Autodesk Fusion 360 part; units mm, degrees
sketch "Sketch1" plane through (0, 0, 0) normal (0, 1, 0) x (1, 0, 0)
  line L0 (20, 0) -> (40, 0)
  line L1 (40, 0) -> (40, -15)
  line L2 (26, -45) -> (0, -45)
  line L3 (-26, -45) -> (0, -45)
  line L4 (-40, 0) -> (-40, -15)
  line L5 (-20, 0) -> (-40, 0)
  line L6 (20, -20) -> (-20, -20)
  line L7 (-20, -20) -> (-20, 0)
  line L8 (20, 0) -> (20, -20)
  line L9 (-40, 0) -> (-40, -15)
  line L10 (0, -45) -> (-26, -45)
  line L11 (-40, -15) -> (-26, -45)
  line L12 (40, -15) -> (26, -45)
  dimension "d5" = 15
  dimension "d6" = 26
extrude "Extrude1" add sketch "Sketch1" along normal mid plane 60
sketch "Sketch3" plane through (0, 0, 0) normal (1, 0, 0) x (0, 1, 0)
  line L0 (-30, 45) -> (-21, 45)
  line L1 (-21, 45) -> (-21, 30)
  line L2 (-21, 30) -> (-30, 30)
  line L3 (-30, 30) -> (-30, 45)
  line L4 (21, 45) -> (21, 30)
  line L5 (21, 30) -> (30, 30)
  line L6 (30, 30) -> (30, 45)
  line L7 (30, 45) -> (21, 45)
  dimension "d9" = 9
  dimension "d10" = 15
extrude "Extrude2" cut sketch "Sketch3" along normal mid plane 120
sketch "Sketch4" plane through (0, 0, 45) normal (0, 0, 1) x (-1, 0, 0)
  line L0 (-26, -21) -> (26, -21)
  line L1 (26, -21) -> (26, 21)
  line L2 (26, 21) -> (-26, 21)
  line L3 (-26, 21) -> (-26, -21)
  line L4 (40, 30) -> (40, 15)
  line L5 (40, 15) -> (50, 15)
  line L6 (50, 15) -> (50, -15)
  line L7 (50, -15) -> (40, -15)
  line L8 (40, -15) -> (28, -15)
  line L9 (28, -15) -> (28, 15)
  line L10 (28, 15) -> (40, 15)
  line L11 (-50, 15) -> (-50, -15)
  line L12 (-50, -15) -> (-40, -15)
  line L13 (-40, -15) -> (-28, -15)
  line L14 (-28, -15) -> (-28, 15)
  line L15 (-28, 15) -> (-40, 15)
  line L16 (-40, 15) -> (-50, 15)
  dimension "d13" = 15
  dimension "d14" = 10
  dimension "d15" = 30
extrude "Extrude3" add sketch "Sketch4" along normal blind 28 from surface at -45 contours L5 L6 L7 L8 L9 L10 | L11 L12 L13 L14 L15 L16
sketch "Sketch5" plane through (0, 0, 45) normal (0, 0, 1) x (-1, 0, 0)
  line L0 (-26, -21) -> (26, -21)
  line L1 (26, -21) -> (26, 21)
  line L2 (26, 21) -> (-26, 21)
  line L3 (-26, 21) -> (-26, -21)
  circle A0 centre (0, 0) radius 15
  dimension "d19" = 30
extrude "Extrude4" add sketch "Sketch5" along normal blind 30 contours A0
sketch "Sketch6" plane through (0, 0, 0) normal (0, 1, 0) x (-1, 0, 0)
  line L0 (-10, 55) -> (-10, 65)
  line L1 (-10, 55) -> (-18, 55)
  line L2 (-18, 55) -> (-18, 65)
  line L3 (-18, 65) -> (-10, 65)
  line L4 (-10, 65) -> (-10, 55)
  line L5 (18, 55) -> (18, 65)
  line L6 (10, 55) -> (18, 55)
  line L7 (10, 65) -> (10, 55)
  line L8 (18, 65) -> (10, 65)
extrude "Extrude5" cut sketch "Sketch6" along normal mid plane 60
The model under review builds one solid part; all positions refer to its coordinate system, in mm. A direction names the side the tool comes from. Round coordinates to 2 decimals unless told otherwise and drop trailing zeros. Order: outer loops, then holes, each group sorted by start corner. A loop starts at its lowest first (then second) coordinate and runs counter-clockwise, first axis right, second up. Notation, with made-up numbers: (26, 12.25) - (52, 12.25) arc R26 ccw to (52, 38.25) - close; hole circle Ø2 at (-26.75, 74). An arc over 180 degrees is marked (long way). Use one line per item in the form item = value.
Q1. Add section A-A on z = 7. Give the boundary of the cut face in (x, y), then the cut area to 3 significant figures.
Response values:
outline = (-50, -15) - (-40, -15) - (-40, -30) - (-20, -30) - (-20, 30) - (-40, 30) - (-40, 15) - (-50, 15) - close; (20, -30) - (40, -30) - (40, -15) - (50, -15) - (50, 15) - (40, 15) - (40, 30) - (20, 30) - close
area = 3,000 mm^2
Q2. Add section B-B on y = -19. Give the boundary of the cut face in (x, z).
Response values:
outline = (-40, 0) - (-20, 0) - (-20, 20) - (20, 20) - (20, 0) - (40, 0) - (40, 15) - (26, 45) - (-26, 45) - (-40, 15) - close
Q3. Clearance check with flat-ended pins moving along their axes: P1, Ø6, axis at y = -20.5, z = 45.5, coming from the +X side; P2, Ø12, axis at y = -16, z = 38, coming from the +X side; P3, Ø5, axis at x = -42.5, y = -4.5, coming from the +Z side. State where each tip first meets the part, or that it passes through.
Response values:
P1 = 27.17
P2 = 32.07
P3 = 28
Q4. Tool access review of faces 1 (the flat face through (-10, 0, 60)), 2 (the flat face through (0, -25, 30)), 3 (the flat face through (42, 0, 28)): name each direction out of +Z, -Z, +X, -X, +Y, -Y from which nothing blocks a thin tool from reaching the whole face with its end or side.
Response values:
face_1 = -X, +Y, -Y
face_2 = +Z, +X, -X, -Y
face_3 = +Z, +X, +Y, -Y
Q5. Add section D-D on z = 63. Give the boundary of the cut face in (x, y).
Response values:
outline = (-10, -11.18) arc R15 ccw to (10, -11.18) - (10, 11.18) arc R15 ccw to (-10, 11.18) - close
Q6. Mouldability with a two-part tool opening along X and no side actions: class faces 4 (the flat face through (-31, 0, 0)), 5 (the flat face through (-40, -23, 7)), 6 (the flat face through (-20, 0, 10)) as pulls with the +X half, pulls with the -X half, needs draft (parallel to the pull), parting line crosses it, or undercut.
Response values:
face_4 = needs draft
face_5 = pulls with the -X half
face_6 = undercut
Q7. To check wall thickness, follow line 1 (Z direction, x = 11, y = 9); line 2 (X direction, y = -0.5, z = 13.5); line 3 (Y direction, x = -22, z = 41.5). State the ranges of each line that lie inside material, in increasing order.
Response values:
line_1 = 20 to 55, 65 to 75
line_2 = -50 to -20, 20 to 50
line_3 = -21 to 21
Q8. Add section C-C on x = 0. Give the boundary of the cut face in (y, z), then the cut area to 3 significant figures.
Response values:
outline = (-30, 20) - (30, 20) - (30, 30) - (21, 30) - (21, 45) - (15, 45) - (15, 75) - (-15, 75) - (-15, 45) - (-21, 45) - (-21, 30) - (-30, 30) - close
area = 2,130 mm^2
